Study the drawing (mm; zero at the part's minimum x, y, z) and answer. A direction names the side the tool comes from. Round coordinates to 2 decimals unless told otherwise and drop trailing zeros. Write each loop counter-clockwise with the first axis right and the second up, starting at its lowest first coordinate (ties: lowest second). Pieces come first, ordered by that corner, then holes. Notation, with made-up numbers: M 37,24.25 L 54,24.25 A33 ccw 54,52.25 Z; hole C 51.5,82 d1. An arc over 180 degrees is marked long. Write each question's results on one line, items separated by ' | '.
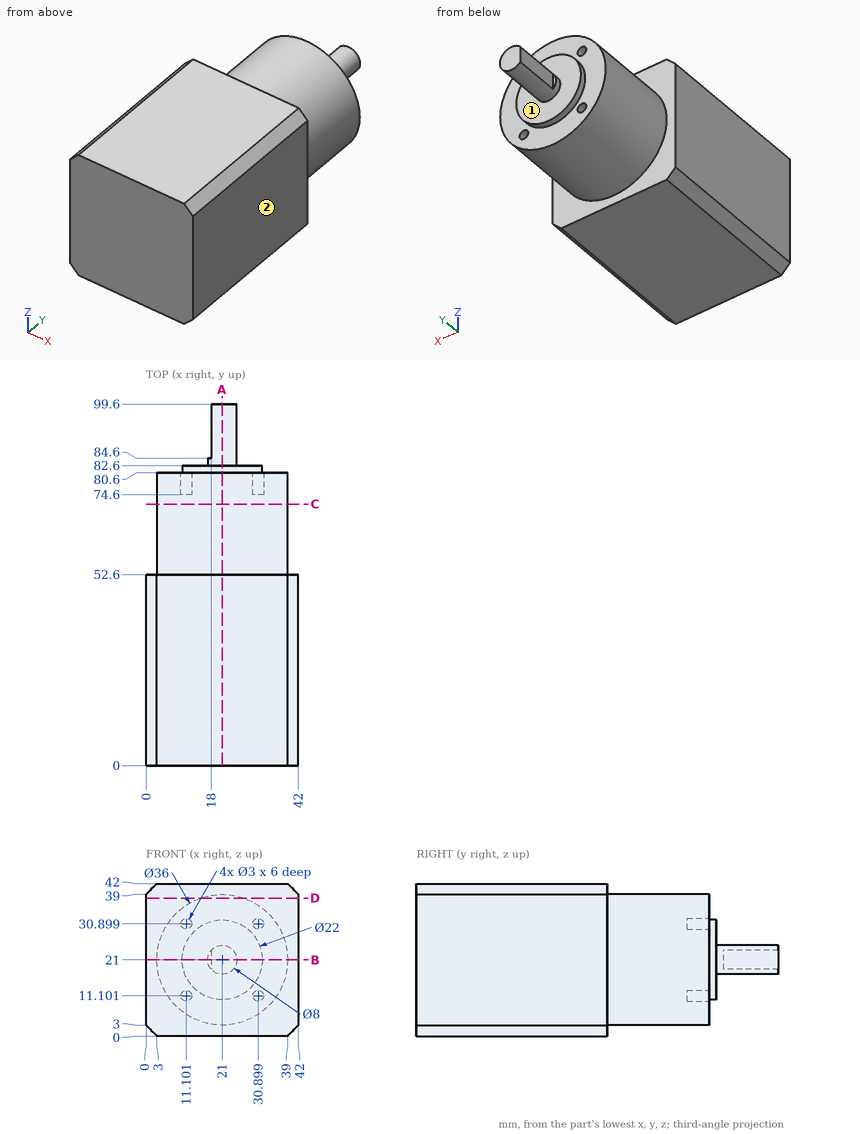
1) Each of these flat-tipped pins is pushed along its axis until it touches: pin 1 (2.5 mm diameter, centred on x = 30.9, z = 11.1, fed in from +Y); pin 2 (1.5 mm diameter, centred on y = 69.5, z = 20.5, fed in from +X); pin 3 (6 mm diameter, centred on x = 16.5, z = 37.5, fed in from +Y). Where does it stop, or does it pass through?
Return value:
pin 1: y = 74.6 | pin 2: x = 39 | pin 3: y = 80.6
2) Find the intervals of material crossed by line 1 (Y direction, x = 13, z = 8.5); line 2 (Y direction, x = 13.5, z = 28.5); line 3 (X direction, y = 57.5, z = 20.5), in increasing order.
Return value:
line 1: 0 to 80.6 | line 2: 0 to 82.6 | line 3: 3.01 to 38.99
3) Section D-D (z = 38) is taken. Determine the outline of the cut face in (x, y), then the cut area to 3 significant figures.
Return value:
outline: M 0,0 L 42,0 L 42,52.6 L 26.92,52.6 L 26.92,80.6 L 15.08,80.6 L 15.08,52.6 L 0,52.6 Z | area: 2,540 mm²
4) Section B-B (z = 21) is taken. Determine the outline of the cut face in (x, y), then the cut area to 3 significant figures.
Return value:
outline: M 0,0 L 42,0 L 42,52.6 L 39,52.6 L 39,80.6 L 32,80.6 L 32,82.6 L 25,82.6 L 25,99.6 L 18,99.6 L 18,84.6 L 17,84.6 L 17,82.6 L 10,82.6 L 10,80.6 L 3,80.6 L 3,52.6 L 0,52.6 Z | area: 3,380 mm²
5) Section C-C (y = 72) is taken. Determine the outline of the cut face in (x, z).
Return value:
outline: C 21,21 d36
6) Section A-A (x = 21) is taken. Determine the outline of the cut face in (y, z).
Return value:
outline: M 0,0 L 52.6,0 L 52.6,3 L 80.6,3 L 80.6,10 L 82.6,10 L 82.6,17 L 99.6,17 L 99.6,25 L 82.6,25 L 82.6,32 L 80.6,32 L 80.6,39 L 52.6,39 L 52.6,42 L 0,42 Z
7) A tool of negligible diameter and unlimited length cuts with its end or side. For the marked faces 1 and 2, from which of +Z, -Z, +X, -X, +Y, -Y can it reach the whole face along a straight path? Write none if from no direction.
Return value:
face 1: +Y | face 2: +Z, -Z, +X, +Y, -Y
